Design review of the part built by this model. Coordinates are the model's own, in mm. Coordinates: 2 decimals unless noted, no trailing zeros. Write each loop counter-clockwise with the first axis right and the second up, starting at its lowest first coordinate (ties: lowest second). Pieces come first, ordered by that corner, then holes. Notation, with made-up numbers: (88, 10) - (101, 10) arc R25 cw to (101, 47) - close; hole circle Ø6 at (16.5, 73). An arc over 180 degrees is marked (long way). Answer as a JSON object with one key per item and string values.
```python
from build123d import *

# Parameters (mm, degrees)
SKETCH1_R           = 5
BOSS_EXTRUDE1_DEPTH = 2.1
SKETCH5_W           = 8.5
SKETCH5_H           = 170.25
BOSS_EXTRUDE3_DEPTH = 6.4
CUT_EXTRUDE2_DEPTH  = 2.1
SKETCH7_W           = 10
SKETCH7_H           = 2.5
BOSS_EXTRUDE4_DEPTH = 3
CHAMFER1_SIZE       = 0.5
SKETCH8_W           = 89.4
SKETCH8_H           = 20
CUT_EXTRUDE3_DEPTH  = 9.5
SKETCH9_R           = 1.75
BOSS_EXTRUDE8_DEPTH = 2.1


with BuildPart() as part:
    # Sketch1 → Boss-Extrude1 (new body)
    with BuildSketch(Plane(origin=(0, 0, 0), x_dir=(1, 0, 0), z_dir=(0, 1, 0))):
        Polygon((-48.95, -172.25), (-48.95, -8), (-42.85, -8), (-40.540598923, -4), (-2.414101615, -4), (4.514101615, 0), (40.640598923, 0), (42.95, 4), (48.95, 4), (48.95, -7.35), (48.95, -165.25), (-40.45, -165.25), (-40.45, -172.25), align=None)
        with Locations((1.05, -100.25)):
            Circle(SKETCH1_R, mode=Mode.SUBTRACT)
        with BuildLine():
            Line((-27.171825407, -133.421572875), (-8.819153161, -115.06890063))
            ThreePointArc((-8.819153161, -115.06890063), (-6.796732371, -113.979375), (-4.508467924, -114.182100859))
            ThreePointArc((-4.508467924, -114.182100859), (1.05, -115.25), (6.608467924, -114.182100859))
            ThreePointArc((6.608467924, -114.182100859), (8.896732371, -113.979375), (10.919153161, -115.06890063))
            Line((10.919153161, -115.06890063), (29.271825407, -133.421572875))
            ThreePointArc((29.271825407, -133.421572875), (30.138916412, -137.780733729), (26.443398282, -140.25))
            Line((26.443398282, -140.25), (-24.343398282, -140.25))
            ThreePointArc((-24.343398282, -140.25), (-28.038916412, -137.780733729), (-27.171825407, -133.421572875))
        make_face(mode=Mode.SUBTRACT)
        with BuildLine():
            Line((-34.95, -9), (-22.556601718, -9))
            ThreePointArc((-22.556601718, -9), (-18.861083588, -11.469266271), (-19.728174593, -15.828427125))
            Line((-19.728174593, -15.828427125), (-32.121572875, -28.221825407))
            ThreePointArc((-32.121572875, -28.221825407), (-36.480733729, -29.088916412), (-38.95, -25.393398282))
            Line((-38.95, -25.393398282), (-38.95, -13))
            ThreePointArc((-38.95, -13), (-37.778427125, -10.171572875), (-34.95, -9))
        make_face(mode=Mode.SUBTRACT)
        with BuildLine():
            Line((41.05, -13), (41.05, -25.393398282))
            ThreePointArc((41.05, -25.393398282), (38.580733729, -29.088916412), (34.221572875, -28.221825407))
            Line((34.221572875, -28.221825407), (21.828174593, -15.828427125))
            ThreePointArc((21.828174593, -15.828427125), (20.961083588, -11.469266271), (24.656601718, -9))
            Line((24.656601718, -9), (37.05, -9))
            ThreePointArc((37.05, -9), (39.878427125, -10.171572875), (41.05, -13))
        make_face(mode=Mode.SUBTRACT)
        with BuildLine():
            Line((-32.121572875, -128.471825407), (-13.76890063, -110.119153161))
            ThreePointArc((-13.76890063, -110.119153161), (-12.679375, -108.096732371), (-12.882100859, -105.808467924))
            ThreePointArc((-12.882100859, -105.808467924), (-13.95, -100.25), (-12.882100859, -94.691532076))
            ThreePointArc((-12.882100859, -94.691532076), (-12.679375, -92.403267629), (-13.76890063, -90.380846839))
            Line((-13.76890063, -90.380846839), (-32.121572875, -72.028174593))
            ThreePointArc((-32.121572875, -72.028174593), (-36.480733729, -71.161083588), (-38.95, -74.856601718))
            Line((-38.95, -74.856601718), (-38.95, -125.643398282))
            ThreePointArc((-38.95, -125.643398282), (-36.480733729, -129.338916412), (-32.121572875, -128.471825407))
        make_face(mode=Mode.SUBTRACT)
        with BuildLine():
            Line((34.221572875, -128.471825407), (15.86890063, -110.119153161))
            ThreePointArc((15.86890063, -110.119153161), (14.779375, -108.096732371), (14.982100859, -105.808467924))
            ThreePointArc((14.982100859, -105.808467924), (16.05, -100.25), (14.982100859, -94.691532076))
            ThreePointArc((14.982100859, -94.691532076), (14.779375, -92.403267629), (15.86890063, -90.380846839))
            Line((15.86890063, -90.380846839), (34.221572875, -72.028174593))
            ThreePointArc((34.221572875, -72.028174593), (38.580733729, -71.161083588), (41.05, -74.856601718))
            Line((41.05, -74.856601718), (41.05, -125.643398282))
            ThreePointArc((41.05, -125.643398282), (38.580733729, -129.338916412), (34.221572875, -128.471825407))
        make_face(mode=Mode.SUBTRACT)
        with BuildLine():
            Line((10.919153161, -85.43109937), (29.271825407, -67.078427125))
            ThreePointArc((29.271825407, -67.078427125), (30.138916412, -62.719266271), (26.443398282, -60.25))
            Line((26.443398282, -60.25), (-24.343398282, -60.25))
            ThreePointArc((-24.343398282, -60.25), (-28.038916412, -62.719266271), (-27.171825407, -67.078427125))
            Line((-27.171825407, -67.078427125), (-8.819153161, -85.43109937))
            ThreePointArc((-8.819153161, -85.43109937), (-6.796732371, -86.520625), (-4.508467924, -86.317899141))
            ThreePointArc((-4.508467924, -86.317899141), (1.05, -85.25), (6.608467924, -86.317899141))
            ThreePointArc((6.608467924, -86.317899141), (8.896732371, -86.520625), (10.919153161, -85.43109937))
        make_face(mode=Mode.SUBTRACT)
        with BuildLine():
            Line((-27.171825407, -33.171572875), (-10.202325554, -16.202073022))
            ThreePointArc((-10.202325554, -16.202073022), (-8.02311566, -15.083537139), (-5.600446128, -15.445131695))
            ThreePointArc((-5.600446128, -15.445131695), (1.05, -17), (7.700446128, -15.445131695))
            ThreePointArc((7.700446128, -15.445131695), (10.12311566, -15.083537139), (12.302325554, -16.202073022))
            Line((12.302325554, -16.202073022), (29.271825407, -33.171572875))
            ThreePointArc((29.271825407, -33.171572875), (30.138916412, -37.530733729), (26.443398282, -40))
            Line((26.443398282, -40), (-24.343398282, -40))
            ThreePointArc((-24.343398282, -40), (-28.038916412, -37.530733729), (-27.171825407, -33.171572875))
        make_face(mode=Mode.SUBTRACT)
        with BuildLine():
            Line((-36.825, -48), (-11.45, -48))
            ThreePointArc((-11.45, -48), (-9.325, -50.125), (-11.45, -52.25))
            Line((-11.45, -52.25), (-36.825, -52.25))
            ThreePointArc((-36.825, -52.25), (-38.95, -50.125), (-36.825, -48))
        make_face(mode=Mode.SUBTRACT)
        with BuildLine():
            Line((13.55, -48), (38.925, -48))
            ThreePointArc((38.925, -48), (41.05, -50.125), (38.925, -52.25))
            Line((38.925, -52.25), (13.55, -52.25))
            ThreePointArc((13.55, -52.25), (11.425, -50.125), (13.55, -48))
        make_face(mode=Mode.SUBTRACT)
    extrude(amount=BOSS_EXTRUDE1_DEPTH)

    # Sketch5 → Boss-Extrude3 (add)
    with BuildSketch(Plane.XZ):
        with Locations((-44.7, 87.125)):
            Rectangle(SKETCH5_W, SKETCH5_H)
    extrude(amount=BOSS_EXTRUDE3_DEPTH)

    # Sketch6 → Cut-Extrude2 (cut)
    with BuildSketch(Plane.ZY.offset(48.95)):
        Polygon((8, 0), (2, 0), (2, -6.4), (145.35, -6.4), (145.35, 0), (140.25, 0), align=None)
    extrude(amount=-CUT_EXTRUDE2_DEPTH, mode=Mode.SUBTRACT)

    # Sketch7 → Boss-Extrude4 (add)
    with BuildSketch(Plane.XZ):
        with Locations((21.05, 2)):
            Rectangle(SKETCH7_W, SKETCH7_H)
    extrude(amount=BOSS_EXTRUDE4_DEPTH)

    # Chamfer1
    chamfer1_edges = [part.edges().sort_by_distance(p)[0] for p in [
        (-48.95, 2.1, 90.125),
    ]]
    chamfer(chamfer1_edges, length=CHAMFER1_SIZE)

    # Sketch8 → Cut-Extrude3 (cut, through all)
    with BuildSketch(Plane(origin=(0, 2.1, 0), x_dir=(1, 0, 0), z_dir=(0, 1, 0))):
        with Locations((4.25, -155.25)):
            Rectangle(SKETCH8_W, SKETCH8_H)
    extrude(amount=-CUT_EXTRUDE3_DEPTH, mode=Mode.SUBTRACT)

    # Sketch9 → Boss-Extrude8 (add)
    with BuildSketch(Plane(origin=(0, 2.1, 0), x_dir=(1, 0, 0), z_dir=(0, 1, 0))):
        with BuildLine():
            Line((-11.319316877, -140.25), (13.419316877, -140.25))
            ThreePointArc((13.419316877, -140.25), (9.889226444, -139.10164524), (7.710401395, -136.096153846))
            ThreePointArc((7.710401395, -136.096153846), (1.05, -131.25), (-5.610401395, -136.096153846))
            ThreePointArc((-5.610401395, -136.096153846), (-7.789226444, -139.10164524), (-11.319316877, -140.25))
        make_face()
        with Locations((1.05, -138.25)):
            Circle(SKETCH9_R, mode=Mode.SUBTRACT)
    extrude(amount=-BOSS_EXTRUDE8_DEPTH)


solid = part.part
```
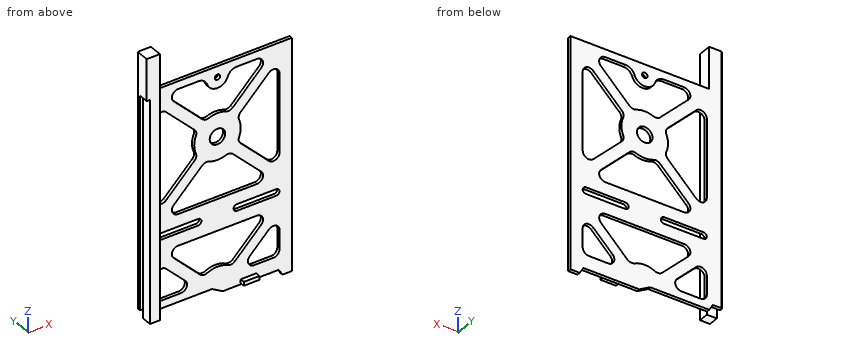
(1) For pin 1 (6 mm diameter, centred on x = 1.05, z = 100.25, fed in from -Y); pin 2 (1.7 mm diameter, centred on x = 26, y = 1.5, fed in from -Z); pin 3 (2 mm diameter, centred on x = -32.5, y = 1, fed in from -Z); pin 4 (1 mm diameter, centred on x = -29, y = 1, fed in from +Z), all flat-tipped, find the tip position at first contact; note any pin that passes through.
Solved:
{"pin 1": "passes through", "pin 2": "stops at z = 0", "pin 3": "stops at z = 4", "pin 4": "stops at z = 145.25"}
(2) Take a section at B-B, the plane z = 138.25. Write out the cut boundary in (x, y), and give its area (3 significant figures).
Solved:
{"outline": "(-48.95, 0) - (-46.85, 0) - (-46.85, -6.4) - (-40.45, -6.4) - (-40.45, 0) - (-27.81, 0) - (-27.81, 2.1) - (-48.45, 2.1) - (-48.95, 1.6) - close; (-6.85, 0) - (-0.7, 0) - (-0.7, 2.1) - (-6.85, 2.1) - close; (2.8, 0) - (8.95, 0) - (8.95, 2.1) - (2.8, 2.1) - close; (29.91, 0) - (48.95, 0) - (48.95, 2.1) - (29.91, 2.1) - close", "area": "151 mm^2"}
(3) To check wall thickness, follow line 1 (X direction, y = 1.35, z = 100.25); line 2 (Z direction, x = -29, y = 0.5); line 3 (Z direction, x = 40, y = 1). State the ranges of each line that lie inside material, in increasing order. Write a range as from..to.
Solved:
{"line 1": "x = -48.95..-38.95, -13.95..-3.95, 6.05..16.05, 41.05..48.95", "line 2": "z = 4..9, 25.1..48, 52.25..75.15, 125.35..145.25", "line 3": "z = 0..10.3, 28.09..48.29, 51.96..72.16, 128.34..145.25"}
(4) Take a section at A-A, the plane x = 1.05. Write out the cut boundary in (y, z).
Solved:
{"outline": "(0, 2) - (2.1, 2) - (2.1, 17) - (0, 17) - close; (0, 40) - (2.1, 40) - (2.1, 60.25) - (0, 60.25) - close; (0, 85.25) - (2.1, 85.25) - (2.1, 95.25) - (0, 95.25) - close; (0, 105.25) - (2.1, 105.25) - (2.1, 115.25) - (0, 115.25) - close; (0, 131.25) - (2.1, 131.25) - (2.1, 136.5) - (0, 136.5) - close; (0, 140) - (2.1, 140) - (2.1, 145.25) - (0, 145.25) - close"}
(5) Take a section at D-D, the plane z = 57.5. Write out the cut boundary in (x, y).
Solved:
{"outline": "(-48.95, 0) - (-46.85, 0) - (-46.85, -6.4) - (-40.45, -6.4) - (-40.45, 0) - (48.95, 0) - (48.95, 2.1) - (-48.45, 2.1) - (-48.95, 1.6) - close"}
(6) Take a section at C-C, the plane y = -4.5. Write out the cut boundary in (x, z).
Solved:
{"outline": "(-48.95, 145.35) - (-46.85, 145.35) - (-46.85, 2) - (-40.45, 2) - (-40.45, 172.25) - (-48.95, 172.25) - close"}
